The model under review builds one solid part; all positions refer to its coordinate system, in mm. A direction names the side the tool comes from. Give positions to 0.01 mm unless a question says otherwise; leave off trailing zeros. Order: outer loops, then holes, each group sorted by start corner. A loop starts at its lowest first (then second) coordinate and runs counter-clockwise, first axis right, second up. Notation, with made-up numbers: (-33.5, 64.5) -> (-0.5, 64.5) arc R24 ccw to (-0.5, 100.5) -> close; hole circle Ø1 at (76, -15.75). An arc over 180 degrees is marked (long way). Answer as a JSON object with one key per item and string values. Group by question number.
from build123d import *

# Parameters (mm, degrees)
BOSS_EXTRUDE1_DEPTH = 20
SKETCH2_W           = 4.5
SKETCH2_H           = 12
CUT_EXTRUDE1_DEPTH  = 17
SKETCH3_R           = 1.5
CUT_EXTRUDE2_DEPTH  = 1
SKETCH3_3_R         = 1.5
CUT_EXTRUDE3_DEPTH  = 7.253189388


with BuildPart() as part:
    # Sketch1 → Boss-Extrude1 (new body)
    with BuildSketch(Plane.XY):
        Polygon((7.5, 9.1), (8.753189388, 9.1), (8.753189388, 7.6), (7.5, 7.6), (7.5, 4.4), (8.753189388, 4.4), (8.753189388, 2.9), (7.5, 2.9), (7.5, 0), (0, 0), (0, 12), (7.5, 12), align=None)
    extrude(amount=BOSS_EXTRUDE1_DEPTH)

    # Sketch2 → Cut-Extrude1 (cut)
    with BuildSketch(Plane.XY.offset(20)):
        with Locations((3.75, 6)):
            Rectangle(SKETCH2_W, SKETCH2_H)
    extrude(amount=-CUT_EXTRUDE1_DEPTH, mode=Mode.SUBTRACT)

    # Sketch3 → Cut-Extrude2 (cut)
    # profile 1 of 6: a face of its own
    with BuildSketch(Plane(origin=(8.753189388, 0, 0), x_dir=(0, 0, -1), z_dir=(1, 0, 0))):
        with BuildLine():
            Line((-5.700961894, 7.6), (-3.42788578, 7.6))
            ThreePointArc((-3.42788578, 7.6), (-3.35, 8.35), (-3.42788578, 9.1))
            Line((-3.42788578, 9.1), (-5.700961894, 9.1))
            ThreePointArc((-5.700961894, 9.1), (-5.551111261, 8.738228568), (-5.5, 8.35))
            ThreePointArc((-5.5, 8.35), (-5.551111261, 7.961771432), (-5.700961894, 7.6))
        make_face()
    # profile 2 of 6: a face of its own
    with BuildSketch(Plane(origin=(8.753189388, 0, 0), x_dir=(0, 0, -1), z_dir=(1, 0, 0))):
        with BuildLine():
            ThreePointArc((-10.57211422, 9.1), (-10.65, 8.35), (-10.57211422, 7.6))
            Line((-10.57211422, 7.6), (-8.299038106, 7.6))
            ThreePointArc((-8.299038106, 7.6), (-8.5, 8.35), (-8.299038106, 9.1))
            Line((-8.299038106, 9.1), (-10.57211422, 9.1))
        make_face()
    # profile 3 of 6: a face of its own
    with BuildSketch(Plane(origin=(8.753189388, 0, 0), x_dir=(0, 0, -1), z_dir=(1, 0, 0))):
        with BuildLine():
            ThreePointArc((-9.792848009, 6), (-7, 0), (-4.207151991, 6))
            ThreePointArc((-4.207151991, 6), (-3.718508564, 6.751777876), (-3.42788578, 7.6))
            Line((-3.42788578, 7.6), (-5.700961894, 7.6))
            ThreePointArc((-5.700961894, 7.6), (-7, 6.85), (-8.299038106, 7.6))
            Line((-8.299038106, 7.6), (-10.57211422, 7.6))
            ThreePointArc((-10.57211422, 7.6), (-10.281491436, 6.751777876), (-9.792848009, 6))
        make_face()
        with Locations((-7, 3.65)):
            Circle(SKETCH3_R, mode=Mode.SUBTRACT)
    # profile 4 of 6: a face of its own
    with BuildSketch(Plane(origin=(8.753189388, 0, 0), x_dir=(0, 0, -1), z_dir=(1, 0, 0))):
        with BuildLine():
            Line((-5.700961894, 9.1), (-3.42788578, 9.1))
            ThreePointArc((-3.42788578, 9.1), (-7, 12), (-10.57211422, 9.1))
            Line((-10.57211422, 9.1), (-8.299038106, 9.1))
            ThreePointArc((-8.299038106, 9.1), (-7, 9.85), (-5.700961894, 9.1))
        make_face()
    # profile 5 of 6: a face of its own
    with BuildSketch(Plane(origin=(8.753189388, 0, 0), x_dir=(0, 0, -1), z_dir=(1, 0, 0))):
        with BuildLine():
            Line((-5.700961894, 7.6), (-3.42788578, 7.6))
            ThreePointArc((-3.42788578, 7.6), (-3.35, 8.35), (-3.42788578, 9.1))
            Line((-3.42788578, 9.1), (-5.700961894, 9.1))
            ThreePointArc((-5.700961894, 9.1), (-5.551111261, 8.738228568), (-5.5, 8.35))
            ThreePointArc((-5.5, 8.35), (-5.551111261, 7.961771432), (-5.700961894, 7.6))
        make_face()
    # profile 6 of 6: a face of its own
    with BuildSketch(Plane(origin=(8.753189388, 0, 0), x_dir=(0, 0, -1), z_dir=(1, 0, 0))):
        with BuildLine():
            ThreePointArc((-10.57211422, 9.1), (-10.65, 8.35), (-10.57211422, 7.6))
            Line((-10.57211422, 7.6), (-8.299038106, 7.6))
            ThreePointArc((-8.299038106, 7.6), (-8.5, 8.35), (-8.299038106, 9.1))
            Line((-8.299038106, 9.1), (-10.57211422, 9.1))
        make_face()
    extrude(amount=-CUT_EXTRUDE2_DEPTH, mode=Mode.SUBTRACT)

    # Sketch3<3> → Cut-Extrude3 (cut)
    with BuildSketch(Plane(origin=(8.753189388, 0, 0), x_dir=(0, 0, -1), z_dir=(1, 0, 0))):
        with BuildLine():
            Line((-8.299038106, 7.6), (-5.700961894, 7.6))
            ThreePointArc((-5.700961894, 7.6), (-5.551111261, 7.961771432), (-5.5, 8.35))
            ThreePointArc((-5.5, 8.35), (-5.551111261, 8.738228568), (-5.700961894, 9.1))
            Line((-5.700961894, 9.1), (-8.299038106, 9.1))
            ThreePointArc((-8.299038106, 9.1), (-8.5, 8.35), (-8.299038106, 7.6))
        make_face()
        with BuildLine():
            ThreePointArc((-8.299038106, 7.6), (-7, 6.85), (-5.700961894, 7.6))
            Line((-5.700961894, 7.6), (-8.299038106, 7.6))
        make_face()
        with BuildLine():
            Line((-8.299038106, 9.1), (-5.700961894, 9.1))
            ThreePointArc((-5.700961894, 9.1), (-7, 9.85), (-8.299038106, 9.1))
        make_face()
        with Locations(Location((-7, 3.65, 0), (0, 0, 30))):
            Circle(SKETCH3_3_R)
    extrude(amount=-CUT_EXTRUDE3_DEPTH, mode=Mode.SUBTRACT)


solid = part.part
1. Take a section at B-B on z = 7. Give the boundary of the cut face in (x, y), plus the area to 3 significant figures.
2. Take a section at D-D on y = 11. Give the boundary of the cut face in (x, z).
3. For probe 1 along X at (y, z) = (1.25, 12); probe 2 along Z at (x, y) = (6.65, 3.65); probe 3 along X at (y, z) = (4.25, 11), list the stretches that pass through material, from the lowest coordinate up. Write a range as [from, to].
4. Take a section at A-A on y = 3.65. Give the boundary of the cut face in (x, z).
5. Draft analysis for pull direction Y (two halves, no side actions). For faces 6 (the flat face through (8.753, 8, 2)), 7 (the flat face through (8, 2.9, 2)), 8 (the flat face through (8, 9.1, 2)), 9 (the flat face through (8, 7.6, 2)), state which applies: pulls with the +Y half, pulls with the -Y half, needs draft (parallel to the pull), parting line crosses it, or undercut.
6. Machinability: for faces 1 (the flat face through (8.753, 8, 15)), 2 (the cylindrical face through (6.89, 2.96, 8.33)), 3 (the flat face through (7.5, 1, 10)), 4 (the flat face through (6, 6, 12)), 5 (the flat face through (8, 4.4, 15)), which of the approach directions +Z, -Z, +X, -X, +Y, -Y give a long, thin tool a straight path to every point of the face, cutting with its end or side? Answer none if there is none.
7. For pin 1 (1.4 mm diameter, centred on x = 8.5, z = 17, fed in from -Y); pin 2 (1 mm diameter, centred on y = 1.5, z = 4, fed in from +X); pin 3 (0.5 mm diameter, centred on y = 4, z = 9, fed in from +X), all flat-tipped, find the tip position at first contact; note any pin that passes through.
8. Take a section at C-C on z = 16.5. Give the boundary of the cut face in (x, y).
Checks:
{
 "1": {"outline": "(0, 0) -> (1.5, 0) -> (1.5, 12) -> (0, 12) -> close; (6, 0) -> (7.5, 0) -> (7.5, 2.15) -> (6, 2.15) -> close; (6, 5.15) -> (7.5, 5.15) -> (7.5, 6.85) -> (6, 6.85) -> close; (6, 9.85) -> (7.5, 9.85) -> (7.5, 12) -> (6, 12) -> close", "area": "27.0 mm2"},
 "2": {"outline": "(0, 0) -> (7.5, 0) -> (7.5, 20) -> (6, 20) -> (6, 3) -> (1.5, 3) -> (1.5, 20) -> (0, 20) -> close"},
 "3": {"probe 1": "x = [0, 1.5], [6, 7.5]", "probe 2": "z = [0, 5.5], [8.5, 20]", "probe 3": "x = [0, 1.5], [6, 8.75]"},
 "4": {"outline": "(0, 0) -> (8.75, 0) -> (8.75, 3.35) -> (7.75, 3.35) -> (7.75, 5.5) -> (6, 5.5) -> (6, 3) -> (1.5, 3) -> (1.5, 20) -> (0, 20) -> close; (6, 8.5) -> (7.75, 8.5) -> (7.75, 10.65) -> (8.75, 10.65) -> (8.75, 20) -> (6, 20) -> close"},
 "5": {"face 6": "needs draft", "face 7": "pulls with the -Y half", "face 8": "pulls with the +Y half", "face 9": "undercut"},
 "6": {"face 1": "+Z, -Z, +X, +Y, -Y", "face 2": "+X", "face 3": "+Z, -Z, +X, -Y", "face 4": "+Z, +Y, -Y", "face 5": "+Z, -Z, +X"},
 "7": {"pin 1": "stops at y = 2.9", "pin 2": "stops at x = 7.5", "pin 3": "stops at x = 7.75"},
 "8": {"outline": "(0, 0) -> (1.5, 0) -> (1.5, 12) -> (0, 12) -> close; (6, 0) -> (7.5, 0) -> (7.5, 2.9) -> (8.75, 2.9) -> (8.75, 4.4) -> (7.5, 4.4) -> (7.5, 7.6) -> (8.75, 7.6) -> (8.75, 9.1) -> (7.5, 9.1) -> (7.5, 12) -> (6, 12) -> close"}
}
